Design review of the part built by this model. Coordinates are the model's own, in mm. Face numbers are marked on the shaded views. Give positions to 0.01 mm unless a question says otherwise; leave off trailing zeros. Loops run counter-clockwise (first coordinate to the right, second up) from the corner with the lowest first, then second, coordinate; pieces in that order, holes last. Notation, with made-up numbers: M 19,-17.75 L 39,-17.75 A33 cw 39,20.25 Z; hole C 20.5,-19 d4. An arc over 180 degrees is marked long. Answer as CSV lines item,"result".
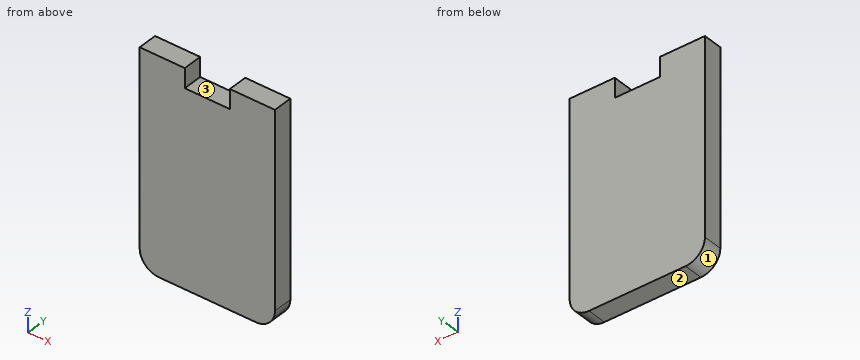
```python
from build123d import *

# Parameters (mm, degrees)
SKETCH2_W           = 21
SKETCH2_H           = 33
BOSS_EXTRUDE1_DEPTH = 3
SKETCH4_W           = 7
SKETCH4_H           = 3
CUT_EXTRUDE2_DEPTH  = 3
FILLET1_R           = 3
FILLET2_R           = 3


with BuildPart() as part:
    # Sketch2 → Boss-Extrude1 (new body)
    with BuildSketch(Plane(origin=(0, 0, 0), x_dir=(1, 0, 0), z_dir=(0, 1, 0))):
        Rectangle(SKETCH2_W, SKETCH2_H)
    extrude(amount=BOSS_EXTRUDE1_DEPTH)

    # Sketch4 → Cut-Extrude2 (cut)
    with BuildSketch(Plane(origin=(0, 3, 0), x_dir=(1, 0, 0), z_dir=(0, 1, 0))):
        with Locations((0, -15)):
            Rectangle(SKETCH4_W, SKETCH4_H)
    extrude(amount=-CUT_EXTRUDE2_DEPTH, mode=Mode.SUBTRACT)

    # Fillet1
    fillet1_edges = [part.edges().sort_by_distance(p)[0] for p in [
        (-10.5, 1.5, -16.5),
    ]]
    fillet(fillet1_edges, radius=FILLET1_R)

    # Fillet2
    fillet2_edges = [part.edges().sort_by_distance(p)[0] for p in [
        (10.5, 1.5, -16.5),
    ]]
    fillet(fillet2_edges, radius=FILLET2_R)


solid = part.part
```
1. We need section A-A, the plane z = 14.5. Write out the cut boundary in (x, y).
Answer block:
outline,"M -10.5,0 L -3.5,0 L -3.5,3 L -10.5,3 Z; M 3.5,0 L 10.5,0 L 10.5,3 L 3.5,3 Z"
2. For P1, Ø0.9, axis at x = 1, y = 1.5, coming from the +Z side, flat-tipped, find the tip position at first contact; note if it passes through.
Answer block:
P1,"z = 13.5"
3. We need section B-B, the plane y = 2.3. Write out the cut boundary in (x, z), plus the area to 3 significant figures.
Answer block:
outline,"M -10.5,-13.5 A3 ccw -7.5,-16.5 L 7.5,-16.5 A3 ccw 10.5,-13.5 L 10.5,16.5 L 3.5,16.5 L 3.5,13.5 L -3.5,13.5 L -3.5,16.5 L -10.5,16.5 Z"
area,"668 mm²"
4. We need section C-C, the plane x = 3. Write out the cut boundary in (y, z).
Answer block:
outline,"M 0,-16.5 L 3,-16.5 L 3,13.5 L 0,13.5 Z"
5. The part is to be moulded in two halves that separate along X. For the marked faces 1, 2 and 3, say which applies: pulls with the +X half, pulls with the -X half, needs draft (parallel to the pull), parting line crosses it, or undercut.
Answer block:
face 1,"pulls with the -X half"
face 2,"needs draft"
face 3,"undercut"
6. To check wall thickness, follow L1, parallel to Z at x = -2.5, y = 1.8; L2, parallel to Z at x = 9.5, y = 0.2. State the ranges of each line that lie inside material, in increasing order. Write a range as [from, to].
Answer block:
L1,"[-16.5, 13.5]"
L2,"[-15.74, 16.5]"
